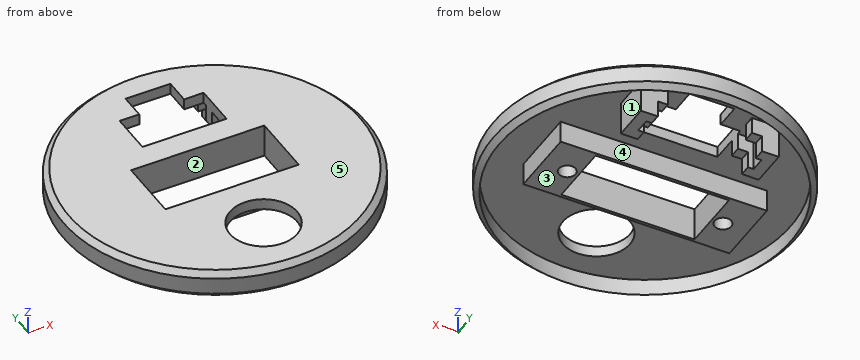
Autodesk Fusion 360 part; units mm, degrees
sketch "Boceto1" plane through (0, 0, 0) normal (0, 0, 1) x (1, 0, 0)
  circle A0 centre (0, 0) radius 27
  dimension "d1" = 54
extrude "Extruir1" add sketch "Boceto1" along normal blind 5
sketch "Boceto2" plane through (0, 0, 0) normal (0, 0, -1) x (1, 0, 0)
  circle A0 centre (0, 0) radius 27
  circle A1 centre (0, 0) radius 26
  dimension "d6" = 52
extrude "Extruir2" cut sketch "Boceto2" against normal blind 3 contours A1
sketch "Boceto3" plane through (0, 0, 5) normal (0, 0, 1) x (-1, 0, 0)
  circle A0 centre (0, 0) radius 27
  line L0 (-11.4, 5.15) -> (11.4, 5.15)
  line L1 (11.4, 5.15) -> (11.4, -5.15)
  line L2 (11.4, -5.15) -> (-11.4, -5.15)
  line L3 (-11.4, -5.15) -> (-11.4, 5.15)
  line L4 (-11.4, 5.15) -> (11.4, -5.15) construction
  line L5 (11.4, 5.15) -> (-11.4, -5.15) construction
  line L6 (0, -27) -> (0, 27) construction
  line L7 (0, 5.15) -> (0, 16) construction
  circle A1 centre (0, 16) radius 6
  dimension "d9" = 10.3
  dimension "d10" = 22.8
  dimension "d11" = 12
extrude "Extruir3" cut sketch "Boceto3" against normal blind 3 contours L0 L1 L2 L3 | A1
sketch "Boceto4" plane through (0, 0, 3) normal (0, 0, -1) x (1, 0, 0)
  circle A0 centre (0, 16) radius 6
  line L0 (-11.4, -5.15) -> (-11.4, 5.15)
  line L1 (-11.4, 5.15) -> (11.4, 5.15)
  line L2 (11.4, 5.15) -> (11.4, -5.15)
  line L3 (11.4, -5.15) -> (-11.4, -5.15)
  circle A1 centre (0, 0) radius 26
  line L4 (-12.4, 6.15) -> (12.4, 6.15)
  line L5 (12.4, 6.15) -> (12.4, -6.15)
  line L6 (12.4, -6.15) -> (-12.4, -6.15)
  line L7 (-12.4, -6.15) -> (-12.4, 6.15)
  line L8 (-12.4, 6.15) -> (12.4, -6.15) construction
  line L9 (12.4, 6.15) -> (-12.4, -6.15) construction
  dimension "d14" = 24.8
  dimension "d15" = 12.3
extrude "Extruir4" add sketch "Boceto4" along normal blind 4 contours L4 L5 L6 L7
chamfer "Chaflán1" distance 1 angle 45 1 edges at (-25.1728, -9.7636, 5)
extrude "Extruir5" add 1 faces at (12.4, -2.05, 0.3333) along direction (1, 0, 0) blind 5
extrude "Extruir6" add 1 faces at (-12.4, 2.05, 0.3333) along direction (-1, 0, 0) blind 5
extrude "Extruir7" add 1 faces at (17.4, -2.05, 0.3333) along direction (1, 0, 0) blind 1
extrude "Extruir8" add 1 faces at (-17.4, 2.05, 0.3333) along direction (-1, 0, 0) blind 1
chamfer "Chaflán2" distance 1 angle 45 1 edges at (-25.1728, -9.7636, 0)
sketch "Boceto5" plane through (0, 0, 5) normal (0, 0, 1) x (-1, 0, 0)
  line L0 (11.4, 5.15) -> (11.4, -5.15)
  line L1 (11.4, -5.15) -> (-11.4, -5.15)
  line L2 (-11.4, -5.15) -> (-11.4, 5.15)
  line L3 (-11.4, 5.15) -> (11.4, 5.15)
  circle A0 centre (0, 16) radius 6
  circle A1 centre (0, 0) radius 26
  line L4 (0, 0) -> (0, -16)
  line L5 (7.5, -10) -> (-7.5, -10)
  line L6 (-7.5, -10) -> (-7.5, -22)
  line L7 (-7.5, -22) -> (7.5, -22)
  line L8 (7.5, -22) -> (7.5, -10)
  line L9 (7.5, -10) -> (-7.5, -22) construction
  line L10 (-7.5, -10) -> (7.5, -22) construction
  line L11 (-7.5, -10) -> (-7.5, -17.5)
  line L12 (-7.5, -17.5) -> (7.5, -17.5)
  line L13 (0, -17.5) -> (-4, -17.5)
  line L14 (-4, -17.5) -> (-4, -22)
  line L15 (-4, -22) -> (4, -22)
  line L16 (4, -22) -> (4, -17.5)
  point P0 (0, -16)
  dimension "d28" = 16
  dimension "d29" = 15
  dimension "d30" = 12
  dimension "d31" = 7.5
extrude "Extruir9" cut sketch "Boceto5" against normal blind 2 contours L5 L6 L8 L11 L12 L13 | L7 L12 L13 L14 L15 L16
sketch "Boceto6" plane through (0, 0, 3) normal (0, 0, -1) x (1, 0, 0)
  line L0 (-4, -17.5) -> (-7.5, -17.5)
  line L1 (-7.5, -17.5) -> (-7.5, -10)
  line L2 (-7.5, -10) -> (7.5, -10)
  line L3 (7.5, -10) -> (7.5, -17.5)
  line L4 (7.5, -17.5) -> (4, -17.5)
  line L5 (4, -17.5) -> (4, -22)
  line L6 (4, -22) -> (-4, -22)
  line L7 (-4, -22) -> (-4, -17.5)
  line L8 (-18.4, 6.15) -> (18.4, 6.15)
  line L9 (18.4, 6.15) -> (18.4, -6.15)
  line L10 (18.4, -6.15) -> (-18.4, -6.15)
  line L11 (-18.4, -6.15) -> (-18.4, 6.15)
  circle A0 centre (0, 16) radius 6
  circle A1 centre (0, 0) radius 26
  line L12 (4, -22) -> (4, -19)
  line L13 (0, -19) -> (10, -19)
  line L14 (10.3, -19.3) -> (10.3, -16.7)
  line L15 (-10.3, -16.7) -> (10.3, -16.7)
  line L16 (-10.3, -19.3) -> (-10.3, -16.7)
  line L17 (10.3, -19.3) -> (-10.3, -19.3)
  line L18 (12.3, -21.3) -> (12.3, -14.7)
  line L19 (-12.3, -14.7) -> (12.3, -14.7)
  line L20 (-12.3, -21.3) -> (-12.3, -14.7)
  line L21 (12.3, -21.3) -> (-12.3, -21.3)
  dimension "d35" = -2
extrude "Extruir10" add sketch "Boceto6" along normal blind 3 contours L1 L7 L15 L16 L17 L19 L20 L21 | L3 L5 L12 L14 L15 L17 L18 L19 L21
sketch "Boceto7" plane through (0, 0, 0) normal (0, 0, -1) x (1, 0, 0)
  line L0 (7.5, -14.7) -> (7.5, -16.7)
  line L1 (7.5, -16.7) -> (10.3, -16.7)
  line L2 (10.3, -16.7) -> (10.3, -19.3)
  line L3 (10.3, -19.3) -> (4, -19.3)
  line L4 (4, -19.3) -> (4, -21.3)
  line L5 (4, -21.3) -> (12.3, -21.3)
  line L6 (12.3, -21.3) -> (12.3, -14.7)
  line L7 (12.3, -14.7) -> (7.5, -14.7)
  line L8 (4, -19.3) -> (7.5002, -19.3)
  line L9 (7.5002, -19.3) -> (7.5002, -21.3)
  line L10 (7.5002, -21.3) -> (4, -21.3)
  line L11 (4, -21.3) -> (4, -19.3)
extrude "Extruir11" cut sketch "Boceto7" against normal blind 3 contours L3 L4 L5 L8 L9 L10 L11
sketch "Boceto8" plane through (0, 0, 0) normal (0, 0, -1) x (1, 0, 0)
  line L0 (-12.3, -21.3) -> (-4, -21.3)
  line L1 (-4, -21.3) -> (-4, -19.3)
  line L2 (-4, -19.3) -> (-10.3, -19.3)
  line L3 (-10.3, -19.3) -> (-10.3, -16.7)
  line L4 (-10.3, -16.7) -> (-7.5, -16.7)
  line L5 (-7.5, -16.7) -> (-7.5, -14.7)
  line L6 (-7.5, -14.7) -> (-12.3, -14.7)
  line L7 (-12.3, -14.7) -> (-12.3, -21.3)
  line L8 (-4, -21.3) -> (-7.5, -21.3)
  line L9 (-7.5, -21.3) -> (-7.5, -19.3)
  line L10 (-7.5, -19.3) -> (-4, -19.3)
  line L11 (-4, -19.3) -> (-4, -21.3)
  line L12 (-12.3, -14.7) -> (-10.3, -14.7)
  line L13 (-10.3, -14.7) -> (-10.3, -21.3)
  line L14 (-10.3, -21.3) -> (-12.3, -21.3)
  line L15 (-12.3, -21.3) -> (-12.3, -14.7)
  line L16 (-10.3, -14.7) -> (-9.3, -14.7)
  line L17 (-9.3, -14.7) -> (-9.3, -16.7)
  line L18 (-9.3, -16.7) -> (-10.3, -16.7)
  line L19 (-10.3, -16.7) -> (-10.3, -14.7)
  line L20 (-10.3, -21.3) -> (-9.3, -21.3)
  line L21 (-9.3, -21.3) -> (-9.3, -19.3)
  line L22 (-9.3, -19.3) -> (-10.3, -19.3)
  line L23 (-10.3, -19.3) -> (-10.3, -21.3)
  dimension "d42" = 1
  dimension "d43" = 1
extrude "Extruir12" cut sketch "Boceto8" against normal blind 3 contours L0 L1 L2 L8 L9 L10 L11
extrude "Extruir14" add sketch "Boceto8" along normal blind 3 contours L0 L3 L6 L7 L12 L13 L14 L15 L19 L23 | L0 L2 L13 L20 L21 L22 L23 | L4 L6 L13 L16 L17 L18 L19
sketch "Boceto9" plane through (0, 0, 0) normal (0, 0, -1) x (1, 0, 0)
  line L0 (7.5002, -19.3) -> (7.5002, -21.3)
  line L1 (7.5002, -21.3) -> (12.3, -21.3)
  line L2 (12.3, -21.3) -> (12.3, -14.7)
  line L3 (12.3, -14.7) -> (7.5, -14.7)
  line L4 (7.5, -14.7) -> (7.5, -16.7)
  line L5 (7.5, -16.7) -> (10.3, -16.7)
  line L6 (10.3, -16.7) -> (10.3, -19.3)
  line L7 (10.3, -19.3) -> (7.5002, -19.3)
  line L8 (12.3, -14.7) -> (9.3, -14.7)
  line L9 (9.3, -14.7) -> (9.3, -16.7)
  line L10 (9.3, -16.7) -> (12.3, -16.7)
  line L11 (12.3, -16.7) -> (12.3, -14.7)
  line L12 (12.3, -21.3) -> (9.3, -21.3)
  line L13 (9.3, -21.3) -> (9.3, -19.3)
  line L14 (9.3, -19.3) -> (12.3, -19.3)
  line L15 (12.3, -19.3) -> (12.3, -21.3)
  dimension "d48" = 3
  dimension "d49" = 3
extrude "Extruir15" add sketch "Boceto9" along normal blind 3 contours L1 L2 L7 L12 L13 L14 L15 | L2 L6 L10 L14 | L2 L3 L5 L8 L9 L10 L11
sketch "Boceto10" plane through (0, 0, -1) normal (0, 0, -1) x (1, 0, 0)
  line L0 (11.4, 5.15) -> (11.4, -5.15)
  line L1 (11.4, -5.15) -> (-11.4, -5.15)
  line L2 (-11.4, -5.15) -> (-11.4, 5.15)
  line L3 (-11.4, 5.15) -> (11.4, 5.15)
  line L4 (-18.4, -6.15) -> (18.4, -6.15)
  line L5 (18.4, -6.15) -> (18.4, 6.15)
  line L6 (18.4, 6.15) -> (-18.4, 6.15)
  line L7 (-18.4, 6.15) -> (-18.4, -6.15)
  line L8 (-11.4, 5.15) -> (-16.4, 5.15)
  line L9 (-16.4, 5.15) -> (-16.4, -5.15)
  line L10 (-16.4, -5.15) -> (-11.4, -5.15)
  line L11 (-11.4, -5.15) -> (-11.4, 5.15)
  line L12 (11.4, 5.15) -> (16.4, 5.15)
  line L13 (16.4, 5.15) -> (16.4, -5.15)
  line L14 (16.4, -5.15) -> (11.4, -5.15)
  line L15 (11.4, -5.15) -> (11.4, 5.15)
  circle A0 centre (-13.9, 0) radius 1.5
  circle A1 centre (13.9, 0) radius 1.5
  dimension "d52" = 5
  dimension "d53" = 5
  dimension "d54" = 3
  dimension "d55" = 3
extrude "Extruir16" cut sketch "Boceto10" against normal blind 4 contours A0 | A1
thread "Rosca1"
thread "Rosca2"
sketch "Boceto11" plane through (0, 0, 5) normal (0, 0, 1) x (-1, 0, 0)
  line L0 (7.5, -17.5) -> (4, -17.5)
  line L1 (4, -17.5) -> (4, -22)
  line L2 (4, -22) -> (-4, -22)
  line L3 (-4, -22) -> (-4, -17.5)
  line L4 (-4, -17.5) -> (-7.5, -17.5)
  line L5 (-7.5, -17.5) -> (-7.5, -10)
  line L6 (-7.5, -10) -> (7.5, -10)
  line L7 (7.5, -10) -> (7.5, -17.5)
  line L8 (11.4, 5.15) -> (11.4, -5.15)
  line L9 (11.4, -5.15) -> (-11.4, -5.15)
  line L10 (-11.4, -5.15) -> (-11.4, 5.15)
  line L11 (-11.4, 5.15) -> (11.4, 5.15)
  circle A0 centre (0, 16) radius 6
  circle A1 centre (0, 0) radius 26
  line L12 (11.9, -5.65) -> (-11.9, -5.65)
  line L13 (-11.9, -5.65) -> (-11.9, 5.65)
  line L14 (-11.9, 5.65) -> (11.9, 5.65)
  line L15 (11.9, 5.65) -> (11.9, -5.65)
  dimension "d58" = -0.5
extrude "Extruir17" cut sketch "Boceto11" against normal blind 10 contours L12 L13 L14 L15
extrude "Extruir13" [suppressed]
equation "d1 = Dex"
equation "Dex = 54 mm"
equation "Din = 52 mm"
equation "d6 = Din"
Geometry: final body of the model. Coordinates: model frame, mm. Face numbers are marked on the shaded views. A direction names the side the tool comes from. Coordinates: 2 decimals unless noted, no trailing zeros. Use one line per item in the form item = value.
1) Section B-B (x = 0). State how many separate pieces and enclosed holes the cut face has, then the cut area to 3 significant figures.
Solutions:
separate_pieces = 4
enclosed_holes = 0
area = 45.4 mm^2
2) Set-up query: the marked faces 1, 2 and 3. Return all of +Z, -Z, +X, -X, +Y, -Y with unobstructed straight access to the full face (end or side cutting, diameter ignored); none if empty.
Solutions:
face_1 = -Z
face_2 = +Z, -Z
face_3 = -Z, +X, -X, -Y
3) Ray query, L1, parallel to X at y = 0, z = -0.15; L2, parallel to Y at x = -0.5, z = 0.25; L3, parallel to Y at x = 10, z = 2. Return the intervals inside material, ascending.
Solutions:
L1 = -18.4 to -15.4, -12.4 to -11.9, 11.9 to 12.4, 15.4 to 18.4
L2 = -26.25 to -26, -6.15 to -5.65, 5.65 to 6.15, 26 to 26.25
L3 = -25.08 to -24, -6.15 to -5.65, 5.65 to 6.15, 14.7 to 16.7, 19.3 to 21.3, 24 to 25.08
4) Mould query, pull axis Y, two halves, no side actions, for the marked faces 4 and 5. Classes: +Y half, -Y half, draft (parallel to the pull), parting line (faces both ways), or undercut.
Solutions:
face_4 = undercut
face_5 = draft
5) Pin query (flat end, axial travel): pin 1 (1.3 mm diameter, centred on y = 18.5, z = 1, fed in from -X); pin 2 (1.6 mm diameter, centred on y = 20.5, z = 2, fed in from -X); pin 3 (1.4 mm diameter, centred on x = -9.5, z = 1, fed in from -Y); pin 4 (7 mm diameter, centred on x = 0, y = -16, fed in from +Z). Return the tip coordinate at first contact, or that it passes through.
Solutions:
pin_1 = -20.26
pin_2 = -18.46
pin_3 = -25.53
pin_4 = through
